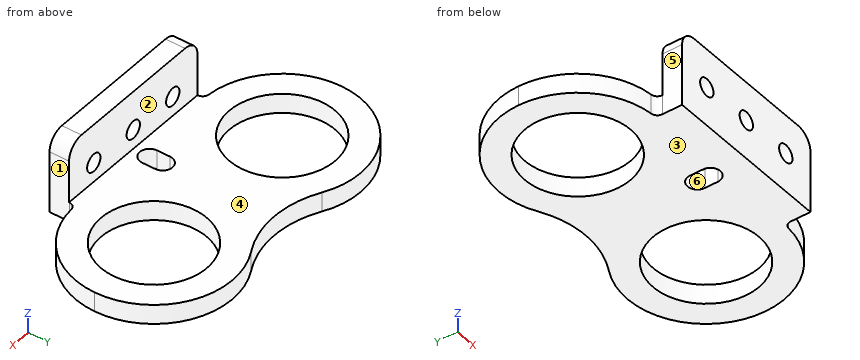
from build123d import *

# Parameters (mm, degrees)
SKETCH1_R           = 8.1
BOSS_EXTRUDE1_DEPTH = 3
SKETCH3_R           = 1.35
BOSS_EXTRUDE2_DEPTH = 3


with BuildPart() as part:
    # Sketch1 → Boss-Extrude1 (new body)
    with BuildSketch(Plane.XY):
        with BuildLine():
            Line((-13, 3.038518603), (-13, 0))
            Line((-13, 0), (13, 0))
            Line((13, 0), (13, 3.038518603))
            ThreePointArc((13, 3.038518603), (13.266200614, 3.717884824), (13.923076923, 4.035555634))
            ThreePointArc((13.923076923, 4.035555634), (21.805592628, 7.847605354), (25, 16))
            ThreePointArc((25, 16), (19.076193076, 26.347940747), (7.153353716, 26.479347653))
            ThreePointArc((7.153353716, 26.479347653), (0, 24.618834191), (-7.153353716, 26.479347653))
            ThreePointArc((-7.153353716, 26.479347653), (-19.076193076, 26.347940747), (-25, 16))
            ThreePointArc((-25, 16), (-21.805592628, 7.847605354), (-13.923076923, 4.035555634))
            ThreePointArc((-13.923076923, 4.035555634), (-13.266200614, 3.717884824), (-13, 3.038518603))
        make_face()
        with BuildLine():
            ThreePointArc((-1.5, 7.5), (0, 9), (1.5, 7.5))
            Line((1.5, 7.5), (1.5, 5.5))
            ThreePointArc((1.5, 5.5), (0, 4), (-1.5, 5.5))
            Line((-1.5, 5.5), (-1.5, 7.5))
        make_face(mode=Mode.SUBTRACT)
        with Locations((-13, 16)):
            Circle(SKETCH1_R, mode=Mode.SUBTRACT)
        with Locations((13, 16)):
            Circle(SKETCH1_R, mode=Mode.SUBTRACT)
    extrude(amount=BOSS_EXTRUDE1_DEPTH)

    # Sketch3 → Boss-Extrude2 (add)
    with BuildSketch(Plane.XZ):
        with BuildLine():
            Line((-13, 3), (13, 3))
            Line((13, 3), (13, 9.5))
            ThreePointArc((13, 9.5), (12.267766953, 11.267766953), (10.5, 12))
            Line((10.5, 12), (-10.5, 12))
            ThreePointArc((-10.5, 12), (-12.267766953, 11.267766953), (-13, 9.5))
            Line((-13, 9.5), (-13, 3))
        make_face()
        with Locations((8, 6)):
            Circle(SKETCH3_R, mode=Mode.SUBTRACT)
        with Locations((-8, 6)):
            Circle(SKETCH3_R, mode=Mode.SUBTRACT)
        with Locations((0, 6)):
            Circle(SKETCH3_R, mode=Mode.SUBTRACT)
    extrude(amount=-BOSS_EXTRUDE2_DEPTH)


solid = part.part
CAD build for the part. Positions are in the model's coordinates, mm. Face numbers are marked on the shaded views. A direction names the side the tool comes from. Give positions to 0.01 mm unless a question says otherwise; leave off trailing zeros. Write each loop counter-clockwise with the first axis right and the second up, starting at its lowest first coordinate (ties: lowest second). Pieces come first, ordered by that corner, then holes. Notation, with made-up numbers: (-23.5, -5.5) -> (-3.5, -5.5) arc R29 cw to (-3.5, 18.5) -> close; hole circle Ø7 at (77.5, -27.75). An arc over 180 degrees is marked (long way). Return JSON: item names as keys, results as strings.
Item 1: Band-saw the part on D-D (x = 10). List the corners of the cut face in (y, z), then the cut area to 3 significant figures.
Answer below:
{"outline": "(0, 0) -> (8.48, 0) -> (8.48, 3) -> (3, 3) -> (3, 12) -> (0, 12) -> close; (23.52, 0) -> (27.62, 0) -> (27.62, 3) -> (23.52, 3) -> close", "area": "64.7 mm2"}
Item 2: Tool access for the marked faces 1, 2 and 3: list every direction of +Z, -Z, +X, -X, +Y, -Y with a clear straight run to the whole face (end or side of a thin tool).
Answer below:
{"face 1": "+Z, -Z, +X, -Y", "face 2": "+Z, +X, -X, +Y", "face 3": "-Z, +X, -X, +Y, -Y"}
Item 3: Two-plate mould, pull along X, no slides. Class the marked faces 4, 5 and 6: +X half, -X half, draft (parallel to the pull), parting line (faces both ways), or undercut.
Answer below:
{"face 4": "draft", "face 5": "-X half", "face 6": "undercut"}
Item 4: Band-saw the part on A-A (x = 0). List the corners of the cut face in (y, z).
Answer below:
{"outline": "(0, 0) -> (4, 0) -> (4, 3) -> (3, 3) -> (3, 4.65) -> (0, 4.65) -> close; (0, 7.35) -> (3, 7.35) -> (3, 12) -> (0, 12) -> close; (9, 0) -> (24.62, 0) -> (24.62, 3) -> (9, 3) -> close"}
Item 5: Drill centre lines: probe 1 along X at (y, z) = (14.5, 2.5); probe 2 along Z at (x, y) = (-8, 2.35); probe 3 along X at (y, z) = (6, 0.5). Where is each one in solid material? Low to high.
Answer below:
{"probe 1": "x = -24.91 to -20.96, -5.04 to 5.04, 20.96 to 24.91", "probe 2": "z = 0 to 4.65, 7.35 to 12", "probe 3": "x = -19.63 to -1.5, 1.5 to 19.63"}
Item 6: Drop flat-ended pins along their axis: pin 1 (7 mm diameter, centred on x = -6, z = 7.5, fed in from +Y); pin 2 (12.5 mm diameter, centred on x = -11.5, y = 12, fed in from +Z); pin 3 (6 mm diameter, centred on x = -15.5, y = 21.5, fed in from -Z); pin 4 (1 mm diameter, centred on y = 6.5, z = 1, fed in from +X). Give the stop position or say it passes through.
Answer below:
{"pin 1": "stops at y = 3", "pin 2": "stops at z = 3", "pin 3": "stops at z = 0", "pin 4": "stops at x = 20.94"}
Item 7: Band-saw the part on C-C (y = 25.5). List the corners of the cut face in (x, z).
Answer below:
{"outline": "(-20.33, 0) -> (-5.01, 0) -> (-5.01, 3) -> (-20.33, 3) -> close; (5.01, 0) -> (20.33, 0) -> (20.33, 3) -> (5.01, 3) -> close"}
Item 8: Band-saw the part on B-B (z = 1.25). List the corners of the cut face in (x, y), then the cut area to 3 significant figures.
Answer below:
{"outline": "(-13.92, 4.04) arc R1 cw to (-13, 3.04) -> (-13, 0) -> (13, 0) -> (13, 3.04) arc R1 cw to (13.92, 4.04) arc R12 ccw (long way) to (7.15, 26.48) arc R14.68 cw to (-7.15, 26.48) arc R12 ccw (long way) to start; hole circle Ø16.2 at (-13, 16); hole (-1.5, 5.5) arc R1.5 ccw to (1.5, 5.5) -> (1.5, 7.5) arc R1.5 ccw to (-1.5, 7.5) -> close; hole circle Ø16.2 at (13, 16)", "area": "710 mm2"}
